```python
from build123d import *

# Parameters (mm, degrees)
F0_W         = 30
F0_H         = 30
F0_W_2       = 24
F0_H_2       = 24
F1_DEPTH     = 100
F3_DEPTH     = 30
F5_DEPTH     = 30
F7_DEPTH     = 6
F9_DEPTH     = 50
F13_W        = 30
F13_H        = 30
F14_DEPTH    = 30
F12_W        = 30
F12_H        = 30
F12_W_2      = 23.9601944461
F12_H_2      = 23.7035881728
F15_DEPTH    = 350
F16_T1_DEPTH = 184.300979278
F18_DEPTH    = 44.18
F19_SIZE     = 5.99
F20_SIZE     = 5.99999


# Not quite as in the source:
# - a fillet or chamfer that OpenCascade refuses, or shapes differently, is made with other operations: its cross-section is extruded or revolved along the edge and cut away or added
# - a fillet or chamfer is up to 0.001 mm smaller than in the source, because OpenCascade refuses the exact size


with BuildPart() as f1:
    # F0 (on Right) → F1 (new body)
    with BuildSketch(Plane.YZ):
        Rectangle(F0_W, F0_H)
        Rectangle(F0_W_2, F0_H_2, mode=Mode.SUBTRACT)
    extrude(amount=F1_DEPTH)

    # F2 (on face) → F3 (cut)
    with BuildSketch(Plane(origin=(0, 15, 0), x_dir=(-1, 0, 0), z_dir=(0, 1, 0))):
        Polygon((0, 15), (-30, -15), (0, -15), align=None)
    extrude(amount=-F3_DEPTH, mode=Mode.SUBTRACT)

    # F4 (on face) → F5 (cut)
    with BuildSketch(Plane.XZ.offset(15)):
        Polygon((70, -15), (100, -15), (100, 15), align=None)
    extrude(amount=-F5_DEPTH, mode=Mode.SUBTRACT)

    # F6 (on face) → F7 (join)
    with BuildSketch(Plane(origin=(42.5, 0, -42.5), x_dir=(0, 1, 0), z_dir=(0.7071067812, 0, -0.7071067812))):
        Polygon((-15, 38.8908729653), (15, 38.8908729653), (15, 43.1335136524), (12, 43.1335136524), (-12, 43.1335136524), (-15, 43.1335136524), align=None)
    extrude(amount=F7_DEPTH)

    # F8 (on face) → F9 (cut, symmetric)
    with BuildSketch(Plane(origin=(27.5, 0, 27.5), x_dir=(0, -1, 0), z_dir=(-0.7071067812, 0, -0.7071067812))):
        with BuildLine():
            ThreePointArc((9.63e-08, -60.1040764009), (9.510586241, -56.1646625738), (13.45, -46.6540764009))
            ThreePointArc((13.45, -46.6540764009), (0, -33.2040764009), (-13.45, -46.6540764009))
            ThreePointArc((-13.45, -46.6540764009), (-9.5105861729, -56.1646626419), (9.63e-08, -60.1040764009))
        make_face()
        with BuildLine():
            Line((13.45, -60.1040764009), (13.45, -46.6540764009))
            ThreePointArc((13.45, -46.6540764009), (9.510586241, -56.1646625738), (9.63e-08, -60.1040764009))
            Line((9.63e-08, -60.1040764009), (13.45, -60.1040764009))
        make_face()
        with BuildLine():
            ThreePointArc((9.63e-08, -60.1040764009), (-9.5105861729, -56.1646626419), (-13.45, -46.6540764009))
            Line((-13.45, -46.6540764009), (-13.45, -60.1040764009))
            Line((-13.45, -60.1040764009), (9.63e-08, -60.1040764009))
        make_face()
    extrude(amount=F9_DEPTH, both=True, mode=Mode.SUBTRACT)

    # F13 (on face) → F14 (cut)
    with BuildSketch(Plane(origin=(0, 15, 0), x_dir=(-1, 0, 0), z_dir=(0, 1, 0))):
        with Locations((-15, 0)):
            Rectangle(F13_W, F13_H)
    extrude(amount=-F14_DEPTH, mode=Mode.SUBTRACT)

    # F12 (on face) → F15 (join)
    with BuildSketch(Plane.YZ.offset(30)):
        Rectangle(F12_W, F12_H)
        with Locations((0.0199027769, -0.1482059136)):
            Rectangle(F12_W_2, F12_H_2, mode=Mode.SUBTRACT)
    extrude(amount=-F15_DEPTH)

    # F16: chamfer of 30 on 1 edges, made by hand

    # F16_s2 → F16_t1 (cut)
    with BuildSketch(Plane.XZ.offset(-92.150489639)):
        Polygon((-290, -15), (-320, 15), (-320, -15), align=None)
    extrude(amount=F16_T1_DEPTH, mode=Mode.SUBTRACT)

    # F17 (on face) → F18 (join)
    with BuildSketch(Plane(origin=(30.5, 0, 30.5), x_dir=(0, 1, 0), z_dir=(0.7071067812, 0, 0.7071067812))):
        Polygon((-13.45, -60.1040764009), (-15, -60.1040764009), (-15, -66.1040764009), (15, -66.1040764009), (15, -60.1040764009), (13.45, -60.1040764009), align=None)
    extrude(amount=F18_DEPTH)

    # F19
    f19_edges = [f1.edges().sort_by_distance(p)[0] for p in [
        (104.239978, 0, 19.239978),
    ]]
    chamfer(f19_edges, length=F19_SIZE)

    # F20 (size 6 in the source; OpenCascade refuses exactly that, so slightly less here)
    f20_edges = [f1.edges().sort_by_distance(p)[0] for p in [
        (74.242641, 0, -19.242641),
    ]]
    chamfer(f20_edges, length=F20_SIZE)


solid = f1.part
```
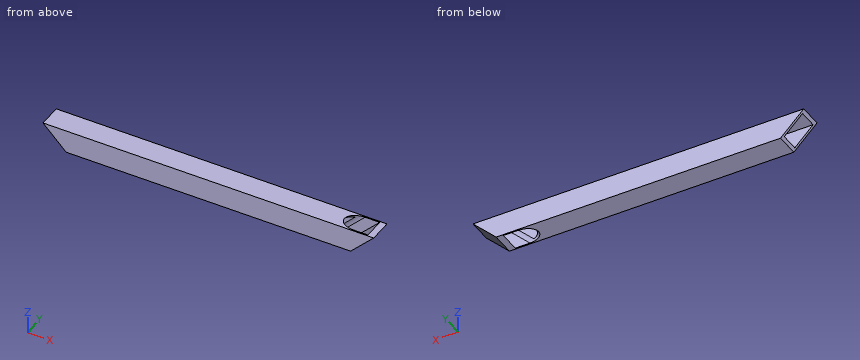
Design review of the part built by this model. Coordinates are the model's own, in mm. Coordinates: 2 decimals unless noted, no trailing zeros. Order: outer loops, then holes, each group sorted by start corner. A loop starts at its lowest first (then second) coordinate and runs counter-clockwise, first axis right, second up. Notation, with made-up numbers: (66, 73) - (81, 73) arc R17 ccw to (81, 95) - close; hole circle Ø8 at (40.25, -10.75). An arc over 180 degrees is marked (long way). One line per question, with ' | ' between items.
Q1. Clearance check with flat-ended pins moving along their axes: pin 1 Ø12 at (y, z) = (0, -7.5) entering from -X; pin 2 Ø8 at (y, z) = (1.5, 9.5) entering from -X; pin 3 Ø1 at (y, z) = (-1, -7.5) entering from -X. State where each tip first meets the part, or that it passes through.
Answer key:
pin 1: stops at x = -293 | pin 2: stops at x = -318.5 | pin 3: stops at x = 77
Q2. To check wall thickness, follow line 1 along Y through (x, z) = (-277, 1); line 2 along Z through (x, y) = (-45, 5); line 3 along Y through (x, z) = (70.5, 6). State the ranges of each line that lie inside material, in increasing order.
Answer key:
line 1: y = -15 to -11.96, 12 to 15 | line 2: z = -15 to -12, 11.7 to 15 | line 3: y = -15 to -13.41, 13.41 to 15
Q3. Consider section A-A, the plane x = -174.5. Give the boundary of the cut face in (y, z), then the cut area to 3 significant figures.
Answer key:
outline: (-15, -15) - (15, -15) - (15, 15) - (-15, 15) - close; hole (-11.96, -12) - (12, -12) - (12, 11.7) - (-11.96, 11.7) - close | area: 332 mm2
Q4. Consider section B-B, the plane y = 6. Give the number of separate pieces and of enclosed holes in the cut face, then the cut area to 3 significant figures.
Answer key:
separate pieces: 3 | enclosed holes: 0 | area: 2,480 mm2
